Can you work these out from the model? Positions are in its coordinate system, mm. Face numbers are marked on the shaded views. A direction names the side the tool comes from. Give positions to 0.01 mm unless a question says otherwise; leave off trailing zeros. Write each loop counter-clockwise with the first axis right and the second up, starting at its lowest first coordinate (ties: lowest second). Pieces come first, ordered by that corner, then holes. Notation, with made-up numbers: (50, 58.5) -> (68, 58.5) arc R15 cw to (68, 74.5) -> close; hole circle Ø9 at (40, -23.75). An arc over 180 degrees is marked (long way). One line per item, written item: value.
Autodesk Fusion 360 part; units mm, degrees
sketch "Sketch1" plane through (0, 0, 0) normal (0, 0, 1) x (1, 0, 0)
  circle A0 centre (0, 0) radius 26.5
  circle A1 centre (0, 0) radius 37.5
  line L0 (-35.6931, 26.5) -> (64.3069, 26.5)
  line L1 (64.3069, 26.5) -> (64.3069, 11.5)
  line L2 (64.3069, 11.5) -> (-35.6931, 11.5)
  line L3 (-35.6931, 11.5) -> (-35.6931, 26.5)
  line L4 (-35.6931, 26.5) -> (64.3069, 26.5)
  line L5 (64.3069, 26.5) -> (64.3069, 56.5)
  line L6 (64.3069, 56.5) -> (-35.6931, 56.5)
  line L7 (-35.6931, 56.5) -> (-35.6931, 26.5)
  circle A2 centre (0, 0) radius 20.5
  line L8 (-23.8747, 11.5) -> (-23.8747, 56.5)
  line L9 (23.8747, 11.5) -> (23.8747, 56.5)
  line L10 (18.4691, 8.8962) -> (23.8747, 11.5)
  line L11 (-23.8747, 11.5) -> (-18.4691, 8.8962)
  dimension "d1" = 53
  dimension "d2" = 75
  dimension "d3" = 100
  dimension "d4" = 15
  dimension "d5" = 30
  dimension "d12" = 41
extrude "Extrude1" add sketch "Sketch1" along normal blind 17 contours A0 A2 L10 L11 | A0 A1 L2 | A1 L0 L2 L4 L9 | A1 L0 L2 L4 L8
extrude "Extrude2" add sketch "Sketch1" along normal blind 6 from surface at 17 contours A0 A2 L10 L11 | A0 A1 L2 | A0 L2 A2 | A1 L0 L2 L4 L9 | L2 A2 L10 | A0 L0 L4 L9 | A0 L0 L4 L8 | A1 L0 L2 L4 L8 | L2 A2 L11 | L2 A2 | L2 A2
extrude "Extrude3" add sketch "Sketch1" against normal blind 10 contours A0 A2 L10 L11
equation "d2 = 53 mm + ( 2 * 11 ) * 1 mm"
equation "d12 = 53 mm - 12 mm"
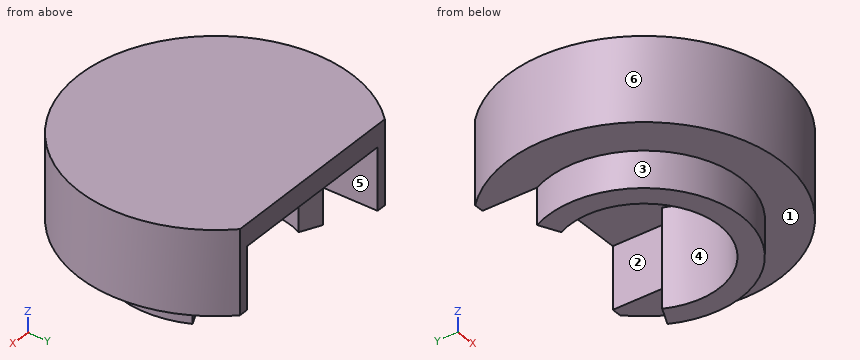
1) Will these pins go through, and if not, where does the flat tip stop? pin 1 (8 mm diameter, centred on x = -27, z = 18, fed in from -Y); pin 2 (4.5 mm diameter, centred on y = 22.5, z = 12, fed in from +X); pin 3 (12 mm diameter, centred on x = -21, z = -5.5, fed in from +Y).
Answer list:
pin 1: stops at y = -29.62
pin 2: stops at x = 31.56
pin 3: stops at y = 11.5
2) For the marked faces 4, 5 and 6, which set-ups out of +Z, -Z, +X, -X, +Y, -Y let a thin tool reach every point of the face, with its end or its side?
Answer list:
face 4: -Z
face 5: -Z, +Y
face 6: +Z, -Z
3) If we section it at B-B (y = 0): Write out the boundary of the cut face in (x, z).
Answer list:
outline: (-37.5, 0) -> (-26.5, 0) -> (-26.5, -10) -> (-20.5, -10) -> (-20.5, 17) -> (20.5, 17) -> (20.5, -10) -> (26.5, -10) -> (26.5, 0) -> (37.5, 0) -> (37.5, 23) -> (-37.5, 23) -> close
4) If we section it at C-C (y = 10): Write out the boundary of the cut face in (x, z).
Answer list:
outline: (-36.14, 0) -> (-24.54, 0) -> (-24.54, -10) -> (-20.76, -10) -> (-20.76, 17) -> (20.76, 17) -> (20.76, -10) -> (24.54, -10) -> (24.54, 0) -> (36.14, 0) -> (36.14, 23) -> (-36.14, 23) -> close
5) If we section it at D-D (x = -16.5): Write out the boundary of the cut face in (y, z), and give its area (3 significant figures).
Answer list:
outline: (-33.67, 0) -> (-20.74, 0) -> (-20.74, -10) -> (-12.17, -10) -> (-12.17, 17) -> (26.5, 17) -> (26.5, 23) -> (-33.67, 23) -> close
area: 812 mm^2
6) I need wall thicknesses on L1, parallel to X at y = 0, z = 6.25; L2, parallel to Z at x = -5, y = 23.5; L3, parallel to X at y = 0, z = -2. Which ranges of each line are inside material? Lowest first, please.
Answer list:
L1: x = -37.5 to -20.5, 20.5 to 37.5
L2: z = 17 to 23
L3: x = -26.5 to -20.5, 20.5 to 26.5
7) We'd pull the mould along X, two halves only. Please class the marked faces 1, 2 and 3: released by +X, released by -X, zero draft, split by the parting line, or undercut.
Answer list:
face 1: zero draft
face 2: undercut
face 3: split by the parting line
8) If we section it at A-A (x = 0): Write out the boundary of the cut face in (y, z).
Answer list:
outline: (-37.5, 0) -> (-26.5, 0) -> (-26.5, -10) -> (-20.5, -10) -> (-20.5, 17) -> (26.5, 17) -> (26.5, 23) -> (-37.5, 23) -> close
